from build123d import *

# Parameters (mm, degrees)
BOSS_EXTRUDE1_DEPTH = 3.175
CUT_EXTRUDE1_DEPTH  = 7.35
CUT_EXTRUDE2_DEPTH  = 7.62


with BuildPart() as part:
    # Sketch1 → Boss-Extrude1 (new body, symmetric)
    with BuildSketch(Plane.XY):
        Polygon((76.2, 37.697541537), (76.2, 56.747541537), (79.375, 56.747541537), (79.375, 37.697541537), (92.075, 37.697541537), (92.075, 46.587541537), (95.25, 46.587541537), (95.25, 37.697541537), (136.525, 37.697541537), (136.525, 46.587541537), (139.7, 46.587541537), (139.7, 37.697541537), (152.4, 37.697541537), (152.4, 69.447541537), (0, 69.447541537), (-0.423998633, 69.491926731), (-3.587863461, 69.757603883), (-946.051908629, 122.953392794), (-946.583462345, 116.623288424), (-943.412318182, 116.444298555), (-943.91275138, 110.48479854), (-6.775989292, 31.791225946), (-5.713280681, 44.446685258), (-2.549415853, 44.181008106), (-3.612124464, 31.525548794), (-1.492292584, 31.347541537), (0, 31.347541537), (0, 44.047541537), (3.175, 44.047541537), (3.175, 31.347541537), (15.875, 31.347541537), (15.875, 36.427541537), (19.05, 36.427541537), (19.05, 31.347541537), (25.4, 31.347541537), (69.85, 37.697541537), align=None)
    extrude(amount=BOSS_EXTRUDE1_DEPTH, both=True)

    # Sketch2 → Cut-Extrude1 (cut, through all)
    with BuildSketch(Plane.XY.offset(3.175)):
        Polygon((-76.254460917, 37.625496217), (-75.245037036, 49.646404609), (-78.411328309, 49.883186), (-79.418325745, 37.891173369), align=None)
        Polygon((-155.224527027, 44.256797945), (-154.27566721, 55.556468134), (-157.441958483, 55.793249525), (-158.388391855, 44.522475098), align=None)
        Polygon((-234.194593137, 50.888099674), (-233.306297384, 61.466531659), (-236.472588657, 61.70331305), (-237.358457965, 51.153776826), align=None)
        Polygon((-313.164659247, 57.519401402), (-312.336927558, 67.376595183), (-315.503218831, 67.613376574), (-316.328524075, 57.785078555), align=None)
        Polygon((-392.134725356, 64.15070313), (-391.367557732, 73.286658708), (-394.533849005, 73.523440099), (-395.298590185, 64.416380283), align=None)
        Polygon((-471.104791466, 70.782004859), (-470.398187906, 79.196722233), (-473.564479179, 79.433503624), (-474.268656294, 71.047682011), align=None)
        Polygon((-550.074857576, 77.413306587), (-549.42881808, 85.106785757), (-552.595109353, 85.343567149), (-553.238722404, 77.67898374), align=None)
        Polygon((-629.044923686, 84.044608316), (-628.459448254, 91.016849282), (-631.625739527, 91.253630673), (-632.208788514, 84.310285468), align=None)
        Polygon((-708.014989796, 90.675910044), (-707.490078428, 96.926912807), (-710.656369701, 97.163694198), (-711.178854624, 90.941587197), align=None)
        Polygon((-786.985055905, 97.307211772), (-786.520708602, 102.836976331), (-789.686999875, 103.073757723), (-790.148920734, 97.572888925), align=None)
        Polygon((-865.955122015, 103.938513501), (-865.551338776, 108.747039856), (-868.717630049, 108.983821247), (-869.118986843, 104.204190653), align=None)
    extrude(amount=-CUT_EXTRUDE1_DEPTH, mode=Mode.SUBTRACT)

    # Sketch3 → Cut-Extrude2 (cut)
    with BuildSketch(Plane.XY.offset(3.175)):
        Polygon((-354.231624716, 60.967890842), (-362.126685184, 71.979397876), (-347.872352174, 77.449083798), (-357.599036746, 89.739165772), (194.218411841, 89.739165772), (127.81181163, -85.755982461), align=None)
    extrude(amount=-CUT_EXTRUDE2_DEPTH, mode=Mode.SUBTRACT)


solid = part.part
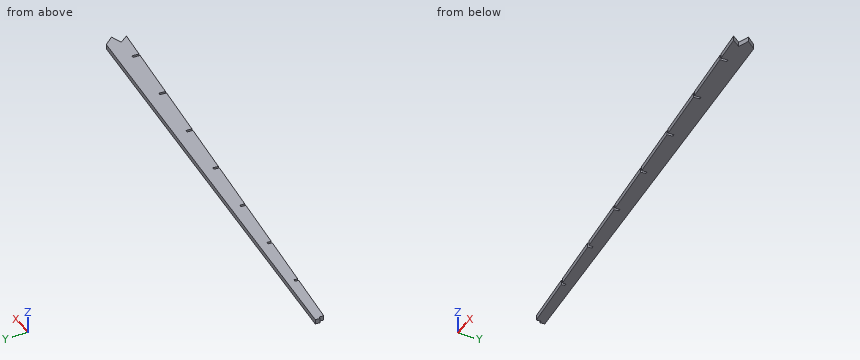
Read the model definition and answer for the solid it produces. Units are mm, in the model's axes. Round coordinates to 2 decimals unless told otherwise and drop trailing zeros. Write each loop counter-clockwise with the first axis right and the second up, starting at its lowest first coordinate (ties: lowest second). Pieces come first, ordered by that corner, then holes. Notation, with made-up numbers: M 3.5,-8.5 L 34.5,-8.5 A18 cw 34.5,19.5 Z; hole C -4.75,35 d4. An arc over 180 degrees is marked long. Use a Markdown table: item, result.
1) The part is cut by section B-B (x = -566). Write down the section's boundary in (y, z) (3 decimals), plus the area to 3 significant figures.
Answers follow:
| item | result |
|---|---|
| outline | M 78.751,-3.175 L 101.502,-3.175 L 101.502,3.175 L 78.751,3.175 Z |
| area | 144 mm2 |
2) Straight lines are drawn through the part: line 1 along Y through (x, z) = (-583.5, 1.75); line 2 along Y through (x, z) = (-752, -1.75). For each, find the intervals that lie inside material, in ascending order. Write a range as [from, to].
Answers follow:
| item | result |
|---|---|
| line 1 | y = [80.22, 102.49] |
| line 2 | y = [94.37, 112] |
3) The part is cut by section A-A (x = -676). Write down the section's boundary in (y, z) (3 decimals), plus the area to 3 significant figures.
Answers follow:
| item | result |
|---|---|
| outline | M 87.988,-3.175 L 107.711,-3.175 L 107.711,3.175 L 87.988,3.175 Z |
| area | 125 mm2 |
4) Flat-ended cylindrical pins translate along their axes: pin 1 (12 mm diameter, centred on x = -570, y = 103.5, fed in from -Z) (3 decimals); pin 2 (2 mm diameter, centred on y = 111, z = -2, fed in from -X). Find the tip coordinate at first contact, or state that the pin passes through.
Answers follow:
| item | result |
|---|---|
| pin 1 | stops at z = -3.175 |
| pin 2 | stops at x = -943.91 |
